The drawing under review shows one solid part. Ordinate dimensions are in mm from its lowest x, y, z. Coordinates: 2 decimals unless noted, no trailing zeros. Write each loop counter-clockwise with the first axis right and the second up, starting at its lowest first coordinate (ties: lowest second). Pieces come first, ordered by that corner, then holes. Notation, with made-up numbers: (-30.75, 43.5) -> (16.25, 43.5) arc R19 cw to (16.25, 72.5) -> close; hole circle Ø9 at (80, 32). An arc over 180 degrees is marked (long way). One line per question, with ' | ' between items. Start each with the question number.
Q1. Add section B-B on x = 5. State the section outline as (y, z) points.
Q2. Add section A-A on z = 5. State the section outline as (x, y) points, and give its area (3 significant figures).
Q3. For P1, Ø1.5, axis at x = 4, z = 8, coming from the +Y side; P2, Ø1.5, axis at x = 8, z = 8, coming from the -Y side, all flat-tipped, find the tip position at first contact; note any pin that passes through.
Q4. Wall thickness on probe 1 along Y at (x, z) = (7.25, 3): over which ranges is the line inside the solid? List them lowest first.
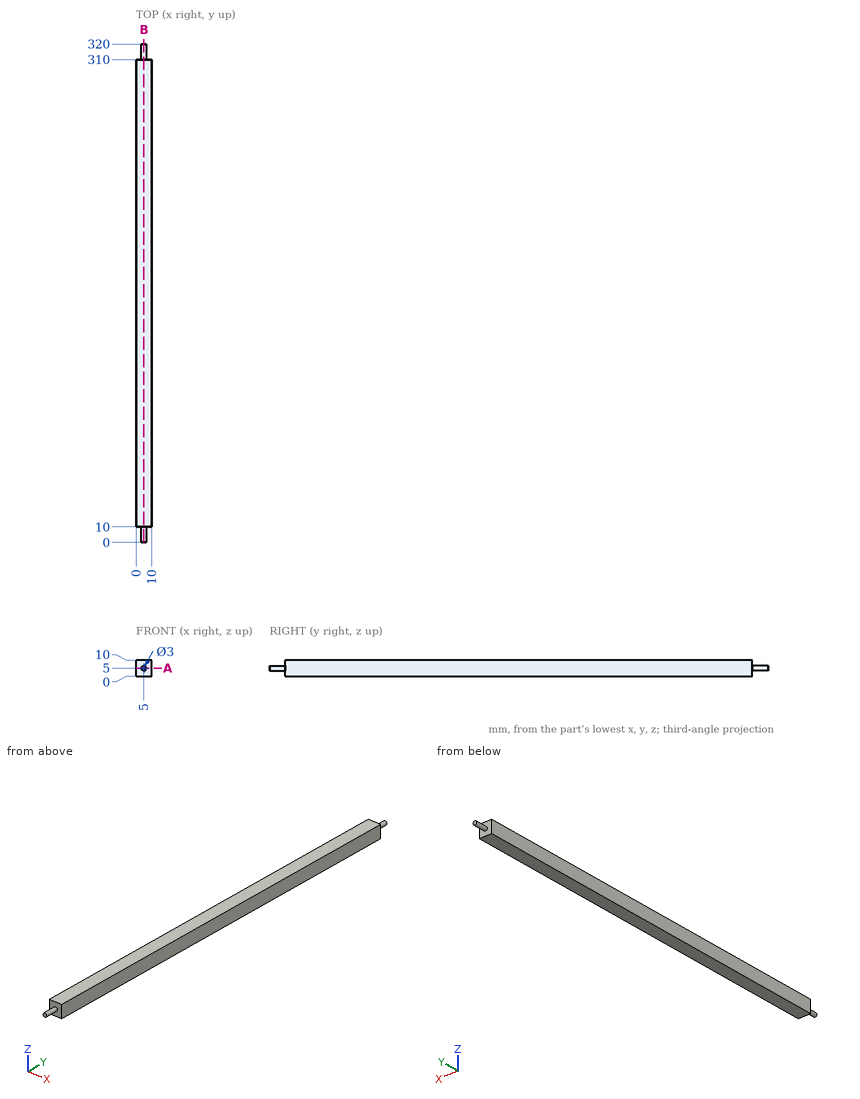
Output values:
1) outline: (0, 3.5) -> (10, 3.5) -> (10, 0) -> (310, 0) -> (310, 3.5) -> (320, 3.5) -> (320, 6.5) -> (310, 6.5) -> (310, 10) -> (10, 10) -> (10, 6.5) -> (0, 6.5) -> close
2) outline: (0, 10) -> (3.5, 10) -> (3.5, 0) -> (6.5, 0) -> (6.5, 10) -> (10, 10) -> (10, 310) -> (6.5, 310) -> (6.5, 320) -> (3.5, 320) -> (3.5, 310) -> (0, 310) -> close | area: 3,060 mm2
3) P1: stops at y = 310 | P2: stops at y = 10
4) probe 1: y = 10 to 310
